Build history of the part. All positions in model axes, mm. Face numbers are marked on the shaded views. A direction names the side the tool comes from. Give positions to 0.01 mm unless a question says otherwise; leave off trailing zeros. Order: outer loops, then holes, each group sorted by start corner. A loop starts at its lowest first (then second) coordinate and runs counter-clockwise, first axis right, second up. Notation, with made-up numbers: (-37, 88) -> (17, 88) arc R15 ccw to (17, 110) -> close; hole circle Ø1 at (40, 17.5). An arc over 180 degrees is marked (long way). Use a Markdown table: item, result. Add a question column.
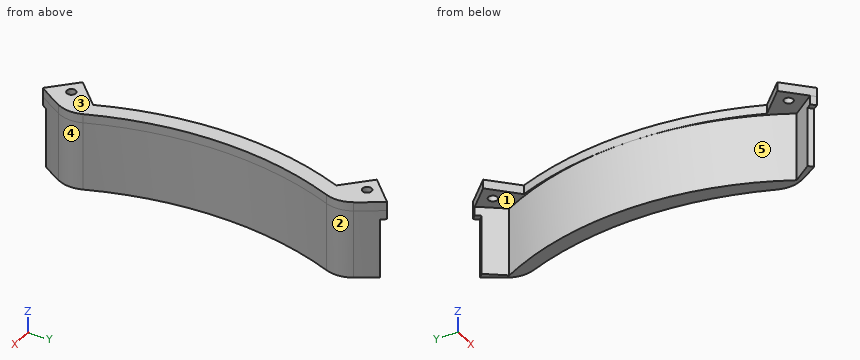
```python
from build123d import *
from build123d.topology import SkipClean

# Parameters (mm, degrees)
CROQUIS1_R              = 100
SALIENTE_EXTRUIR1_DEPTH = 3
CROQUIS3_R              = 110
CORTAR_EXTRUIR1_DEPTH   = 3
REDONDEO1_R             = 10
CORTAR_EXTRUIR6_DEPTH   = 10
CROQUIS12_R             = 1.5
CORTAR_EXTRUIR7_DEPTH   = 142.453172607
CROQUIS9_R              = 1.5
CROQUIS9_W              = 4.5
CROQUIS9_H              = 8
CROQUIS9_W_2            = 8
CROQUIS9_H_2            = 4.5
CORTAR_EXTRUIR5_DEPTH   = 10
CORTAR_EXTRUIR8_DEPTH   = 142.453172607
CROQUIS16_R             = 1.5
CORTAR_EXTRUIR9_DEPTH   = 106.376884656
SALIENTE_EXTRUIR4_DEPTH = 23
SALIENTE_EXTRUIR9_START = 23
SALIENTE_EXTRUIR9_DEPTH = 23
CORTAR_EXTRUIR12_DEPTH  = 20


with BuildPart() as part:
    # Croquis1 → Saliente-Extruir1 (new body)
    with BuildSketch(Plane.XY):
        Circle(CROQUIS1_R)
    extrude(amount=SALIENTE_EXTRUIR1_DEPTH)

    # Croquis3 → Cortar-Extruir1 (cut)
    with BuildSketch(Plane.XY.offset(3)):
        with Locations((190, 0)):
            Circle(CROQUIS3_R)
    extrude(amount=-CORTAR_EXTRUIR1_DEPTH, mode=Mode.SUBTRACT)

    # Redondeo1
    redondeo1_edges = [part.edges().sort_by_distance(p)[0] for p in [
        (89.473684211, -44.659375654, 1.5),
        (89.473684211, 44.659375654, 1.5),
    ]]
    fillet(redondeo1_edges, radius=REDONDEO1_R)

    # Croquis5 → Cortar-Extruir6 (cut)
    with BuildSketch(Plane.XY.offset(3)):
        Polygon((-58.336309448, -83.085046789), (-83.085046789, -58.336309448), (-65.40737726, -40.658639918), (-40.658639918, -65.40737726), align=None)
        Polygon((-83.085046789, 58.336309448), (-58.336309448, 83.085046789), (-40.658639918, 65.40737726), (-65.40737726, 40.658639918), align=None)
        Polygon((58.336309448, -83.085046789), (83.085046789, -58.336309448), (65.40737726, -40.658639918), (40.658639918, -65.40737726), align=None)
        Polygon((58.336309448, 83.085046789), (83.085046789, 58.336309448), (65.40737726, 40.658639918), (40.658639918, 65.40737726), align=None)
    extrude(amount=-CORTAR_EXTRUIR6_DEPTH, mode=Mode.SUBTRACT)

    # Croquis12 → Cortar-Extruir7 (cut, through all)
    with BuildSketch(Plane.XY.offset(3)):
        with Locations((-63.604254904, -36.804908024)):
            Circle(CROQUIS12_R)
        with Locations((-36.804907897, -63.604255031)):
            Circle(CROQUIS12_R)
        with Locations((-47.666068056, -20.866721176)):
            Circle(CROQUIS12_R)
        with Locations((-20.866721049, -47.666068183)):
            Circle(CROQUIS12_R)
        with Locations(Location((47.666068183, 20.866721049, 0), (0, 0, 180))):
            Circle(CROQUIS12_R)
        with Locations(Location((20.866721176, 47.666068056, 0), (0, 0, 180))):
            Circle(CROQUIS12_R)
        with Locations(Location((63.604255031, 36.804907897, 0), (0, 0, 180))):
            Circle(CROQUIS12_R)
        with Locations(Location((36.804908024, 63.604254904, 0), (0, 0, 180))):
            Circle(CROQUIS12_R)
        with Locations((20.866721325, -47.666067908)):
            Circle(CROQUIS12_R)
        with Locations((47.666068332, -20.866720901)):
            Circle(CROQUIS12_R)
        with Locations((63.60425518, -36.804907749)):
            Circle(CROQUIS12_R)
        with Locations((36.804908173, -63.604254756)):
            Circle(CROQUIS12_R)
        with Locations(Location((-63.604254756, 36.804908173, 0), (0, 0, 180))):
            Circle(CROQUIS12_R)
        with Locations(Location((-36.804907749, 63.60425518, 0), (0, 0, 180))):
            Circle(CROQUIS12_R)
        with Locations(Location((-20.866720901, 47.666068332, 0), (0, 0, 180))):
            Circle(CROQUIS12_R)
        with Locations(Location((-47.666067908, 20.866721325, 0), (0, 0, 180))):
            Circle(CROQUIS12_R)
    extrude(amount=-CORTAR_EXTRUIR7_DEPTH, mode=Mode.SUBTRACT)

    # Croquis9 → Cortar-Extruir5 (cut)
    with BuildSketch(Plane.XY.offset(3)):
        with Locations((71.9, -4)):
            Circle(CROQUIS9_R)
        with Locations((35.959143483, 4)):
            Circle(CROQUIS9_R)
        with Locations((71.959143483, 4)):
            Circle(CROQUIS9_R)
        with Locations((35.9, -4)):
            Circle(CROQUIS9_R)
        with Locations((-91.190074744, 4)):
            Circle(CROQUIS9_R)
        with Locations((-91.190074744, -4)):
            Circle(CROQUIS9_R)
        with Locations((-55.190074744, 4)):
            Circle(CROQUIS9_R)
        with Locations((-55.190074744, -4)):
            Circle(CROQUIS9_R)
        with Locations((-4, 85)):
            Circle(CROQUIS9_R)
        with Locations((4, 85)):
            Circle(CROQUIS9_R)
        with Locations((-4, 49)):
            Circle(CROQUIS9_R)
        with Locations((4, 49)):
            Circle(CROQUIS9_R)
        with Locations((-4, -49)):
            Circle(CROQUIS9_R)
        with Locations((4, -49)):
            Circle(CROQUIS9_R)
        with Locations((4, -85)):
            Circle(CROQUIS9_R)
        with Locations((-4, -85)):
            Circle(CROQUIS9_R)
        with Locations((41.209143483, 0)):
            Rectangle(CROQUIS9_W, CROQUIS9_H)
        with Locations((0, -54.25)):
            Rectangle(CROQUIS9_W_2, CROQUIS9_H_2)
        with Locations((-60.440074744, 0)):
            Rectangle(CROQUIS9_W, CROQUIS9_H)
        with Locations((0, 54.25)):
            Rectangle(CROQUIS9_W_2, CROQUIS9_H_2)
    extrude(amount=-CORTAR_EXTRUIR5_DEPTH, mode=Mode.SUBTRACT)

    # Croquis13 → Cortar-Extruir8 (cut, through all)
    with BuildSketch(Plane.XY.offset(3)):
        with BuildLine():
            ThreePointArc((82.185905129, 40.466605039), (74.472042394, 0), (82.185905129, -40.466605039))
            Line((82.185905129, -40.466605039), (73.700623754, -48.951886413))
            Line((73.700623754, -48.951886413), (65.40737726, -40.658639918))
            Line((65.40737726, -40.658639918), (40.658639918, -65.40737726))
            Line((40.658639918, -65.40737726), (57.245132907, -81.993870249))
            ThreePointArc((57.245132907, -81.993870249), (0, -100), (-57.245132907, -81.993870249))
            Line((-57.245132907, -81.993870249), (-40.658639918, -65.40737726))
            Line((-40.658639918, -65.40737726), (-65.40737726, -40.658639918))
            Line((-65.40737726, -40.658639918), (-81.993870249, -57.245132907))
            ThreePointArc((-81.993870249, -57.245132907), (-100, 0), (-81.993870249, 57.245132907))
            Line((-81.993870249, 57.245132907), (-65.40737726, 40.658639918))
            Line((-65.40737726, 40.658639918), (-40.658639918, 65.40737726))
            Line((-40.658639918, 65.40737726), (-57.245132907, 81.993870249))
            ThreePointArc((-57.245132907, 81.993870249), (0, 100), (57.245132907, 81.993870249))
            Line((57.245132907, 81.993870249), (40.658639918, 65.40737726))
            Line((40.658639918, 65.40737726), (65.40737726, 40.658639918))
            Line((65.40737726, 40.658639918), (73.700623754, 48.951886413))
            Line((73.700623754, 48.951886413), (82.185905129, 40.466605039))
        make_face()
    extrude(amount=-CORTAR_EXTRUIR8_DEPTH, mode=Mode.SUBTRACT)

    # Croquis16 → Cortar-Extruir9 (cut, through all)
    with BuildSketch(Plane(origin=(0, 0, 0), x_dir=(-1, 0, 0), z_dir=(0, 0, -1))):
        with Locations((-79.619107513, -49.213515922)):
            Circle(CROQUIS16_R)
        with Locations((-79.620014024, 49.214422433)):
            Circle(CROQUIS16_R)
    extrude(amount=-CORTAR_EXTRUIR9_DEPTH, mode=Mode.SUBTRACT)

    # Croquis17 → Saliente-Extruir4 (add)
    with SkipClean():  # the faces are left unmerged after this step: merging them gives an invalid solid
        with BuildSketch(Plane(origin=(0, 0, 0), x_dir=(-1, 0, 0), z_dir=(0, 0, -1))):
            with BuildLine():
                ThreePointArc((-87.134502924, 49.067080616), (-74.472042394, 0), (-87.134502924, -49.067080616))
                ThreePointArc((-87.134502924, -49.067080616), (-88.3979419, -44.839843317), (-87.719298246, -40.480341508))
                ThreePointArc((-87.719298246, -40.480341508), (-80, 0), (-87.719298246, 40.480341508))
                ThreePointArc((-87.719298246, 40.480341508), (-88.3979419, 44.839843317), (-87.134502924, 49.067080616))
            make_face()
        extrude(amount=SALIENTE_EXTRUIR4_DEPTH)

    # Croquis19 → Saliente-Extruir9 (add)
    with SkipClean():  # the faces are left unmerged after this step: merging them gives an invalid solid
        with BuildSketch(Plane(origin=(0, 0, 0), x_dir=(-1, 0, 0), z_dir=(0, 0, -1)).offset(SALIENTE_EXTRUIR9_START)):
            with BuildLine():
                Line((-81.993870249, -57.245132907), (-80.578491296, -55.829753954))
                Line((-80.578491296, -55.829753954), (-86.470047942, -47.845734499))
                Line((-86.470047942, -47.845734499), (-87.134502924, -49.067080616))
                ThreePointArc((-87.134502924, -49.067080616), (-84.662989481, -53.218213162), (-81.993870249, -57.245132907))
            make_face()
            with BuildLine():
                Line((-81.993870249, 57.245132907), (-80.578491296, 55.829753954))
                Line((-80.578491296, 55.829753954), (-86.470047942, 47.845734499))
                Line((-86.470047942, 47.845734499), (-87.134502924, 49.067080616))
                ThreePointArc((-87.134502924, 49.067080616), (-84.662989481, 53.218213162), (-81.993870249, 57.245132907))
            make_face()
        extrude(amount=-SALIENTE_EXTRUIR9_DEPTH)

    # Croquis21 → Cortar-Extruir12 (cut)
    with SkipClean():  # the faces are left unmerged after this step: merging them gives an invalid solid
        with BuildSketch(Plane(origin=(0, 0, -23), x_dir=(-1, 0, 0), z_dir=(0, 0, -1))):
            with BuildLine():
                Line((-80.578491296, -55.829753954), (-81.768004725, -54.217769392))
                Line((-81.768004725, -54.217769392), (-83.120763907, -55.596210371))
                ThreePointArc((-83.120763907, -55.596210371), (-82.898820117, -56.654058957), (-81.993870249, -57.245132907))
                Line((-81.993870249, -57.245132907), (-80.578491296, -55.829753954))
            make_face()
            with BuildLine():
                Line((-80.578491296, 55.829753954), (-81.768004725, 54.217769392))
                Line((-81.768004725, 54.217769392), (-83.141306562, 55.565485178))
                ThreePointArc((-83.141306562, 55.565485178), (-82.91545484, 56.642950884), (-81.993870249, 57.245132907))
                Line((-81.993870249, 57.245132907), (-80.578491296, 55.829753954))
            make_face()
        extrude(amount=-CORTAR_EXTRUIR12_DEPTH, mode=Mode.SUBTRACT)


solid = part.part
```
(1) Band-saw the part on D-D on y = 26.5. Give the cut face in (x, z).
(2) Band-saw the part on A-A on x = 84.25. Give the cut face in (y, z).
(3) Band-saw the part on B-B on z = -10.75. Give the cut face in (x, y).
(4) Wall check: probe 1 along Z at (x, y) = (81.5, 48); probe 2 along X at (y, z) = (-0.5, 1.75); probe 3 along X at (y, z) = (-32, -5.75). Give the ranges that are in metal, low to high.
(5) Pin check, flat tips, straight feed: pin 1 Ø6 at (y, z) = (3.5, -10) entering from +X; pin 2 Ø5 at (y, z) = (20, -18) entering from +X; pin 3 Ø10 at (y, z) = (-15, -8.5) entering from -X; pin 4 Ø6.5 at (x, y) = (77.5, 34.5) entering from -Z. Stop position of each tip, or through.
(6) Band-saw the part on C-C on x = 75.75. Give the cut face in (y, z), plus the area to 3 significant figures.
(7) Mould opens along Y. For the marked faces 1, 2 and 3 say: released by +Y, released by -Y, zero draft, split by the parting line, or undercut.
(8) Tool access for the marked faces 4 and 5: list every direction of +Z, -Z, +X, -X, +Y, -Y with a clear straight run to the whole face (end or side of a thin tool).
Response:
| question | item | result |
|---|---|---|
| 1 | outline | (77.71, 0) -> (78, 0) -> (78, -23) -> (83.24, -23) -> (83.24, 3) -> (77.71, 3) -> close |
| 2 | outline | (-53.87, -23) -> (-50.85, -23) -> (-50.85, 0) -> (-43.44, 0) -> (-43.44, -23) -> (-30.28, -23) -> (-30.28, 3) -> (-53.87, 3) -> close; (30.28, -23) -> (43.44, -23) -> (43.44, 0) -> (50.85, 0) -> (50.85, -23) -> (53.87, -23) -> (53.87, 3) -> (30.28, 3) -> close |
| 3 | outline | (81.77, -54.22) -> (83.12, -55.6) arc R100 ccw to (87.13, -49.07) arc R10 ccw to (87.72, -40.48) arc R110 cw to (87.72, 40.48) arc R10 ccw to (87.13, 49.07) arc R100 ccw to (83.14, 55.57) -> (81.77, 54.22) -> (86.47, 47.85) arc R101.4 ccw to (86.47, -47.85) -> close |
| 4 | probe 1 | z = 0 to 3 |
| 4 | probe 2 | x = 74.47 to 80 |
| 4 | probe 3 | x = 79.65 to 84.76 |
| 5 | pin 1 | stops at x = 80.19 |
| 5 | pin 2 | stops at x = 82.33 |
| 5 | pin 3 | stops at x = 74.97 |
| 5 | pin 4 | stops at z = -23 |
| 6 | outline | (-51, 0) -> (-46.9, 0) -> (-46.9, 3) -> (-51, 3) -> close; (-16.72, 0) -> (-16.05, 0) -> (-16.05, -23) -> (16.05, -23) -> (16.05, 0) -> (16.72, 0) -> (16.72, 3) -> (-16.72, 3) -> close; (46.9, 0) -> (51, 0) -> (51, 3) -> (46.9, 3) -> close |
| 6 | area | 863 mm² |
| 7 | face 1 | undercut |
| 7 | face 2 | undercut |
| 7 | face 3 | zero draft |
| 8 | face 4 | +Z, -Z, +X |
| 8 | face 5 | -Z, -X |
